Input: part model. Units: mm. Frame: model coordinates. A direction names the side the tool comes from. Coordinates: 2 decimals unless noted, no trailing zeros. Write each loop counter-clockwise with the first axis right and the second up, starting at its lowest first coordinate (ties: lowest second). Pieces come first, ordered by that corner, then holes. Notation, with made-up numbers: (-34.75, -5) - (-3.75, -5) arc R26 ccw to (-3.75, 16) - close; hole circle Ø6 at (62.5, 33.25). An arc over 180 degrees is marked (long way). Use CSV: the item, a comma, the result in double quotes.
```python
from build123d import *
from OCP.BRepAlgoAPI import BRepAlgoAPI_Cut
from OCP.TopTools import TopTools_ListOfShape

# Parameters (mm, degrees)
BOSS_EXTRUDE1_DEPTH = 58
SKETCH1_4_R         = 6
BOSS_EXTRUDE3_DEPTH = 6
CUT_EXTRUDE8_DEPTH  = 26
RIB14_REACH         = 110.472
SKETCH8_WALL_W      = 275.405915094
SKETCH8_WALL_H      = 10
SKETCH10_R          = 10
CUT_EXTRUDE10_DEPTH = 21


with BuildPart() as part:
    # Sketch1 → Boss-Extrude1 (new body)
    with BuildSketch(Plane.XY):
        with BuildLine():
            Line((-18.973896199, 9), (-18.973896199, 0))
            ThreePointArc((-18.973896199, 0), (-13.421880234, -13.411258999), (-0.015020694, -18.973890253))
            ThreePointArc((-0.015020694, -18.973890253), (9.87730883, -23.078310175), (13.973896199, -32.973885866))
            Line((13.973896199, -32.973885866), (13.973896199, -108))
            ThreePointArc((13.973896199, -108), (14.559682636, -109.414213562), (15.973896199, -110))
            Line((15.973896199, -110), (19.973896199, -110))
            Line((19.973896199, -110), (19.973896199, 0))
            Line((19.973896199, 0), (15.848197366, 0))
            ThreePointArc((15.848197366, 0), (14.525476133, -0.499863827), (13.863935397, -1.749591462))
            ThreePointArc((13.863935397, -1.749591462), (-0.876521771, -13.946378905), (-13.973896199, 0))
            Line((-13.973896199, 0), (-13.973896199, 9))
            ThreePointArc((-13.973896199, 9), (-14.559682636, 10.414213562), (-15.973896199, 11))
            Line((-15.973896199, 11), (-16.973896199, 11))
            ThreePointArc((-16.973896199, 11), (-18.388109761, 10.414213562), (-18.973896199, 9))
        make_face()
    extrude(amount=BOSS_EXTRUDE1_DEPTH)

    # Sketch1_4 → Boss-Extrude3 (add)
    with BuildSketch(Plane.XY):
        with BuildLine():
            ThreePointArc((58.366201044, -24.31995715), (54.61491235, -38.31995715), (58.366201044, -52.31995715))
            ThreePointArc((58.366201044, -52.31995715), (59.876313249, -56.792715074), (59.544360912, -61.501834946))
            Line((59.544360912, -61.501834946), (48.544360912, -101.501834946))
            ThreePointArc((48.544360912, -101.501834946), (45.301079262, -106.960444534), (39.726458462, -110))
            Line((39.726458462, -110), (19.973896199, -110))
            Line((19.973896199, -110), (19.973896199, 0))
            Line((19.973896199, 0), (50.505709466, -6.590084108))
            ThreePointArc((50.505709466, -6.590084108), (58.944097052, -13.456348075), (58.366201044, -24.31995715))
        make_face()
        with Locations((36.973896199, -98.31995715)):
            Circle(SKETCH1_4_R, mode=Mode.SUBTRACT)
        with Locations((47.973896199, -58.31995715)):
            Circle(SKETCH1_4_R, mode=Mode.SUBTRACT)
        with Locations((47.973896199, -18.31995715)):
            Circle(SKETCH1_4_R, mode=Mode.SUBTRACT)
    extrude(amount=BOSS_EXTRUDE3_DEPTH)

    # Sketch6 → Cut-Extrude8 (cut)
    with BuildSketch(Plane(origin=(19.973896199, 0, 0), x_dir=(0, 0, -1), z_dir=(1, 0, 0))):
        with BuildLine():
            Line((-40, -40), (-25, -40))
            ThreePointArc((-25, -40), (-20.757359313, -38.242640687), (-19, -34))
            Line((-19, -34), (-19, -26))
            ThreePointArc((-19, -26), (-20.757359313, -21.757359313), (-25, -20))
            Line((-25, -20), (-40, -20))
            ThreePointArc((-40, -20), (-44.242640687, -21.757359313), (-46, -26))
            Line((-46, -26), (-46, -34))
            ThreePointArc((-46, -34), (-44.242640687, -38.242640687), (-40, -40))
        make_face()
    extrude(amount=-CUT_EXTRUDE8_DEPTH, mode=Mode.SUBTRACT)

    # Sketch8 wall → Rib14 (add, up to next)
    with BuildSketch(Plane(origin=(30.973896199, -58.31995715, 32), x_dir=(0.389639990837, 0, -0.920967251069), z_dir=(-0.920967251069, 0, -0.389639990837)), mode=Mode.PRIVATE) as rib14_sk1:
        Rectangle(SKETCH8_WALL_W, SKETCH8_WALL_H)
    rib14_tool1 = extrude(rib14_sk1.sketch, amount=RIB14_REACH, mode=Mode.PRIVATE) - part.part
    add(rib14_tool1.solids().sort_by_distance((30.973896199, -58.31995715, 32))[0])


with BuildPart() as cut_extrude10_tool:
    # Sketch10 → Cut-Extrude10 (new body)
    with BuildSketch(Plane(origin=(19.973896199, 0, 0), x_dir=(0, 0, -1), z_dir=(1, 0, 0))):
        with BuildLine():
            ThreePointArc((-26.000000311, -110), (-37.257208214, -106.531039387), (-44.609335124, -97.327526611))
            Line((-44.609335124, -97.327526611), (-58, -63.31995715))
            Line((-58, -63.31995715), (-58, -110))
            Line((-58, -110), (-26.000000311, -110))
        make_face()
        with Locations((-26, -90)):
            Circle(SKETCH10_R)
    extrude(amount=-CUT_EXTRUDE10_DEPTH)


with BuildPart() as part_1:
    add(part.part)

    # Cut-Extrude10: cut by cut_extrude10_tool, with a tolerance
    cut_extrude10_stock = TopTools_ListOfShape()
    cut_extrude10_stock.Append(part_1.part.wrapped)
    cut_extrude10_tools = TopTools_ListOfShape()
    cut_extrude10_tools.Append(cut_extrude10_tool.part.wrapped)
    cut_extrude10_cut = BRepAlgoAPI_Cut()
    cut_extrude10_cut.SetArguments(cut_extrude10_stock)
    cut_extrude10_cut.SetTools(cut_extrude10_tools)
    cut_extrude10_cut.SetFuzzyValue(0.00001)
    cut_extrude10_cut.Build()
    add(Compound.cast(cut_extrude10_cut.Shape()).solids(), mode=Mode.REPLACE)


solid = part_1.part
```
(1) Reachability of faces 4 (the flat face through (18, 0, 29)), 5 (the flat face through (13.974, -70, 29)), 6 (the cylindrical face through (14.345, -21.711, 44.196)), 7 (the flat face through (28, -63.32, 24)), 8 (the cylindrical face through (53.516, -60.618, 2.958)) from +Z, -Z, +X, -X, +Y, -Y: full face, straight path, thin tool, end or side. Return the list, or none.
Check values:
face 4,"+Z, -Z, +X, +Y"
face 5,"+Z, -Z, -X, -Y"
face 6,"+X, -X"
face 7,"+Z, +X, -Y"
face 8,"+Z, -Z"
(2) Cut plane C-C on x = 35.5. Return loops of the section in (y, z).
Check values:
outline,"(-110, 0) - (-104.14, 0) - (-104.14, 6) - (-110, 6) - close; (-92.5, 0) - (-3.35, 0) - (-3.35, 6) - (-53.32, 6) - (-53.32, 21.3) - (-63.32, 21.3) - (-63.32, 6) - (-92.5, 6) - close"
(3) Cut plane B-B on z = 20.5. Return loops of the section in (x, y).
Check values:
outline,"(-18.97, 0) arc R18.97 ccw to (-0.02, -18.97) arc R14 cw to (8.71, -22.03) - (19.97, -22.03) - (19.97, 0) - (15.85, 0) arc R2 ccw to (13.86, -1.75) arc R13.97 cw to (-13.97, 0) - (-13.97, 9) arc R2 ccw to (-15.97, 11) - (-16.97, 11) arc R2 ccw to (-18.97, 9) - close; (13.97, -108) arc R2 ccw to (15.97, -110) - (19.97, -110) - (19.97, -98.35) - (13.97, -98.35) - close; (13.97, -81.65) - (19.97, -81.65) - (19.97, -63.32) - (35.84, -63.32) - (35.84, -53.32) - (19.97, -53.32) - (19.97, -37.97) - (13.97, -37.97) - close"
(4) Draft query along Z for faces 1 (the flat face through (25, -110, 5)), 2 (the flat face through (30.82, -58.39, 32.36)), 3 (the cylindrical face through (17.016, -38.289, 20.804)). Return one class per face: pulls with the +Z half, pulls with the -Z half, needs draft (parallel to the pull), parting line crosses it, or undercut.
Check values:
face 1,"needs draft"
face 2,"pulls with the +Z half"
face 3,"undercut"
(5) Cut plane D-D on x = 52.5. Return loops of the section in (y, z).
Check values:
outline,"(-87.12, 0) - (-62.26, 0) - (-62.26, 6) - (-87.12, 6) - close; (-54.38, 0) - (-22.26, 0) - (-22.26, 6) - (-54.38, 6) - close; (-14.38, 0) - (-7.21, 0) - (-7.21, 6) - (-14.38, 6) - close"
(6) Cut plane A-A on y = -90. Return loops of the section in (x, z), and give its area (3 significant figures).
Check values:
outline,"(13.97, 0) - (51.71, 0) - (51.71, 6) - (19.97, 6) - (19.97, 16) - (13.97, 16) - close; (13.97, 36) - (19.97, 36) - (19.97, 47.49) - (13.97, 47.49) - close"
area,"355 mm^2"
(7) Pin query (flat end, axial travel): pin 1 Ø12 at (x, z) = (10, 34.5) entering from -Y; pin 2 Ø9.5 at (x, y) = (47.97, -18.32) entering from +Z; pin 3 Ø24 at (x, z) = (34, 30) entering from -Y; pin 4 Ø5 at (x, y) = (32, -67.5) entering from -Z. Return the tip coordinate at first contact, or that it passes through.
Check values:
pin 1,"y = -109.45"
pin 2,"through"
pin 3,"y = -63.32"
pin 4,"z = 0"
(8) Ray query, probe 1 along X at (y, z) = (2.5, 26); probe 2 along X at (y, z) = (-94, 37); probe 3 along Y at (x, z) = (28.5, 7.5). Return the intervals inside material, ascending. Write a range as from..to.
Check values:
probe 1,"-18.97..-13.97"
probe 2,"13.97..19.97"
probe 3,"-63.32..-53.32"
